from build123d import *

# Parameters (mm, degrees)
GE_20327_OUTLINE_R = 3.3782
GE_20327_DEPTH     = 3.175
SKETCH3_W          = 2.921
SKETCH3_H          = 1168.4
CUT_EXTRUDE1_DEPTH = 2144.256699657


# Read off the part's stored shape, not the designer's step: GE-20327
with BuildPart() as part:
    # GE-20327 outline → GE-20327 (new body)
    with BuildSketch(Plane.XY):
        Polygon((1828.8, -50.8), (1828.8, 1117.6), (0, 0), (0, -50.8), align=None)
        with Locations((127, 19.05)):
            Circle(GE_20327_OUTLINE_R, mode=Mode.SUBTRACT)
        with Locations((127, 57.15)):
            Circle(GE_20327_OUTLINE_R, mode=Mode.SUBTRACT)
        with Locations((533.4, 19.05)):
            Circle(GE_20327_OUTLINE_R, mode=Mode.SUBTRACT)
        with Locations((533.4, 57.15)):
            Circle(GE_20327_OUTLINE_R, mode=Mode.SUBTRACT)
        with Locations((1257.3, 19.05)):
            Circle(GE_20327_OUTLINE_R, mode=Mode.SUBTRACT)
        with Locations((1257.3, 57.15)):
            Circle(GE_20327_OUTLINE_R, mode=Mode.SUBTRACT)
        with Locations((1701.8, 19.05)):
            Circle(GE_20327_OUTLINE_R, mode=Mode.SUBTRACT)
        with Locations((1701.8, 57.15)):
            Circle(GE_20327_OUTLINE_R, mode=Mode.SUBTRACT)
        with Locations((1816.1, 77.7875)):
            Circle(GE_20327_OUTLINE_R, mode=Mode.SUBTRACT)
        with Locations((1816.1, 399.520833333)):
            Circle(GE_20327_OUTLINE_R, mode=Mode.SUBTRACT)
        with Locations((1816.1, 721.254166667)):
            Circle(GE_20327_OUTLINE_R, mode=Mode.SUBTRACT)
        with Locations((1816.1, 1042.9875)):
            Circle(GE_20327_OUTLINE_R, mode=Mode.SUBTRACT)
    extrude(amount=GE_20327_DEPTH)

    # Sketch3 → Cut-Extrude1 (cut, through all)
    with BuildSketch(Plane(origin=(1828.8, 0, 0), x_dir=(0, 0, -1), z_dir=(1, 0, 0))):
        with Locations((-1.7145, 533.4)):
            Rectangle(SKETCH3_W, SKETCH3_H)
    extrude(amount=-CUT_EXTRUDE1_DEPTH, mode=Mode.SUBTRACT)


solid = part.part
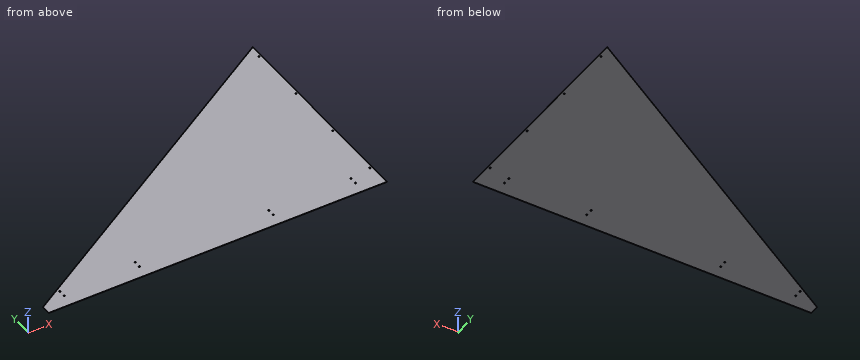
Model file for the job. Use its own axes, mm. Round coordinates to 2 decimals unless told otherwise and drop trailing zeros. Order: outer loops, then holes, each group sorted by start corner. A loop starts at its lowest first (then second) coordinate and runs counter-clockwise, first axis right, second up.
(1) Pin check, flat tips, straight feed: pin 1 (4 mm diameter, centred on x = 1701.8, y = 57.15, fed in from -Z); pin 2 (11 mm diameter, centred on x = 533.4, y = 19.05, fed in from -Z). Stop position of each tip, or through.
(2) Band-saw the part on A-A (x = 1678.5). List the corners of the cut face in (y, z), then the cut area to 3 significant figures.
(3) Band-saw the part on B-B (y = 1016). List the corners of the cut face in (x, z).
(4) Drill centre lines: line 1 (X direction, y = 57.15, z = 0.15); line 2 (Y direction, x = 1816.1, z = 0.2); line 3 (Y direction, x = 533.4, z = 0.2). Where is each one in solid material? Low to high.
Verdict:
1. pin 1: passes through
1. pin 2: stops at z = 0
2. outline: (-50.8, 0) - (1025.75, 0) - (1025.75, 0.25) - (-50.8, 0.25) - close
2. area: 273 mm2
3. outline: (1662.55, 0) - (1828.8, 0) - (1828.8, 0.25) - (1662.55, 0.25) - close
4. line 1: x = 93.52 to 123.62, 130.38 to 530.02, 536.78 to 1253.92, 1260.68 to 1698.42, 1705.18 to 1828.8
4. line 2: y = -50.8 to 74.41, 81.17 to 396.14, 402.9 to 717.88, 724.63 to 1039.61, 1046.37 to 1109.84
4. line 3: y = -50.8 to 15.67, 22.43 to 53.77, 60.53 to 325.97
